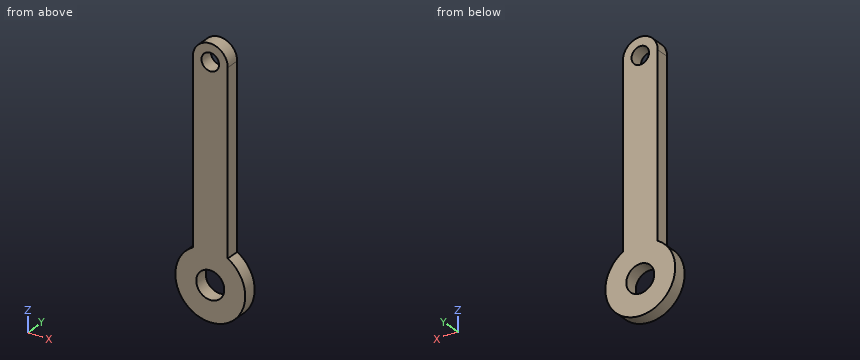
from build123d import *

# Parameters (mm, degrees)
F0_R     = 4
F0_R_2   = 2.5
F1_DEPTH = 4


with BuildPart() as f1:
    # F0 (on Front) → F1 (new body)
    with BuildSketch(Plane.XZ):
        with BuildLine():
            Line((-5, 60), (-5, 8.660254))
            ThreePointArc((-5, 8.660254), (0, -10), (5, 8.660254))
            Line((5, 8.660254), (5, 60))
            ThreePointArc((5, 60), (0, 65), (-5, 60))
        make_face()
        Circle(F0_R, mode=Mode.SUBTRACT)
        with Locations((0, 60)):
            Circle(F0_R_2, mode=Mode.SUBTRACT)
    extrude(amount=F1_DEPTH)


solid = f1.part
Geometry: final body of the model. Coordinates: model frame, mm. Round coordinates to 2 decimals unless told otherwise and drop trailing zeros. Order: outer loops, then holes, each group sorted by start corner. A loop starts at its lowest first (then second) coordinate and runs counter-clockwise, first axis right, second up. Notation, with made-up numbers: (20.25, 48.5) -> (52.25, 48.5) arc R20 ccw to (52.25, 59.5) -> close; hole circle Ø11 at (7, 20). An arc over 180 degrees is marked (long way). Put each result on its own line as item: value. Start each with the question number.
Q1. Section A-A on x = 0. Return the cut outline in (y, z).
Q2. Section D-D on z = 59. Return the cut outline in (x, y), and give its area (3 significant figures).
Q3. Section C-C on y = -0.6. Return the cut outline in (x, z).
Q4. Line query: probe 1 along Z at (x, y) = (0, -2.75); probe 2 along X at (y, z) = (-3.55, 60.5); probe 3 along Z at (x, y) = (-1.5, -3.2). Output: solid intervals per line, ascending.
Q5. Section B-B on z = 0. Return the cut outline in (x, y), and give its area (3 significant figures).
Q6. First-contact query: pin 1 (1.2 mm diameter, centred on y = -1.5, z = 44, fed in from -X); pin 2 (6 mm diameter, centred on x = -7.5, z = 28.5, fed in from +Y); pin 3 (2 mm diameter, centred on x = 5.5, y = -1.5, fed in from +Z). Flat tips, straight axial feed; report the tip coordinate or a pass-through.
Ans:
1. outline: (-4, -10) -> (0, -10) -> (0, -4) -> (-4, -4) -> close; (-4, 4) -> (0, 4) -> (0, 57.5) -> (-4, 57.5) -> close; (-4, 62.5) -> (0, 62.5) -> (0, 65) -> (-4, 65) -> close
2. outline: (-5, -4) -> (-2.29, -4) -> (-2.29, 0) -> (-5, 0) -> close; (2.29, -4) -> (5, -4) -> (5, 0) -> (2.29, 0) -> close
2. area: 21.7 mm2
3. outline: (-5, 8.66) arc R10 ccw (long way) to (5, 8.66) -> (5, 60) arc R5 ccw to (-5, 60) -> close; hole circle Ø8 at (0, 0); hole circle Ø5 at (0, 60)
4. probe 1: z = -10 to -4, 4 to 57.5, 62.5 to 65
4. probe 2: x = -4.97 to -2.45, 2.45 to 4.97
4. probe 3: z = -9.89 to -3.71, 3.71 to 58, 62 to 64.77
5. outline: (-10, -4) -> (-4, -4) -> (-4, 0) -> (-10, 0) -> close; (4, -4) -> (10, -4) -> (10, 0) -> (4, 0) -> close
5. area: 48.0 mm2
6. pin 1: stops at x = -5
6. pin 2: stops at y = 0
6. pin 3: stops at z = 62.18
